The listing builds one solid part. Answer for the finished solid, in the listing's coordinates (mm). A direction names the side the tool comes from. Coordinates: 2 decimals unless noted, no trailing zeros. Loops run counter-clockwise (first coordinate to the right, second up) from the corner with the lowest first, then second, coordinate; pieces in that order, holes last. Notation, with made-up numbers: M 44,7 L 100,7 A30 cw 100,40 Z; hole C 33,-16.75 d2. An arc over 180 degrees is marked long. Answer as a JSON object with one key per item and string values. Group by question number.
1. A cutting plane is placed at C-C on y = 12. Give the vertices of the cut face in (x, z), and give its area (3 significant figures).
2. Straight lines are drawn through the part: L1, parallel to Y at x = 1.75, z = 0; L2, parallel to Z at x = -0.5, y = 17; L3, parallel to Y at x = 4.25, z = -0.5. For each, find the intervals that lie inside material, in ascending order.
3. A cutting plane is placed at D-D on y = -65. Give the vertices of the cut face in (x, z).
4. Given pin 1 (3 mm diameter, centred on y = -21.5, z = 3, fed in from +X); pin 2 (6 mm diameter, centred on x = 3.5, y = -49.5, fed in from -Z); pin 3 (2 mm diameter, centred on x = 4.5, y = 15, fed in from -Z), each flat-ended and moving along its own axis, determine where each tip first touches the part or whether it passes through.
5. Determine the mould class of faces 1 (the face through (0, -75, 0)), 2 (the face through (0, 26, 0)), 3 (the face through (-1.19, -27.12, -5.37)), 4 (the face through (0.054, -63.925, 1.686)) for opening direction Y: released by +Y, released by -Y, zero draft, split by the parting line, or undercut.
6. For faces 5 (the face through (-6.466, 10.353, -2.681)), 6 (the face through (-4, -55, -2)), determine the directions among +Z, -Z, +X, -X, +Y, -Y from which every point of the face is accessible in a straight line to the end or side of a thin tool.
7. A cutting plane is placed at A-A on z = 0. Give the vertices of the cut face in (x, y), and give its area (3 significant figures).
8. A cutting plane is placed at B-B on x = 0. Give the vertices of the cut face in (y, z).
from build123d import *

# Parameters (mm, degrees)
F0_R     = 5.5
F1_DEPTH = 75
F2_R     = 7
F3_DEPTH = 26
F4_SIZE2 = 0.437443
F4_SIZE  = 5
F5_R     = 5.5
F5_R_2   = 4
F6_DEPTH = 20
F7_R     = 2
F8_DEPTH = 12.5


with BuildPart() as f1:
    # F0 (on Front) → F1 (new body)
    with BuildSketch(Plane.XZ):
        Circle(F0_R)
    extrude(amount=F1_DEPTH)

    # F2 (on face) → F3 (join)
    with BuildSketch(Plane(origin=(0, 0, 0), x_dir=(-1, 0, 0), z_dir=(0, 1, 0))):
        Circle(F2_R)
    extrude(amount=F3_DEPTH)

    # F4
    f4_edges = [f1.edges().sort_by_distance(p)[0] for p in [
        (7, 26, 0),
    ]]
    chamfer(f4_edges, length=F4_SIZE, length2=F4_SIZE2)

    # F5 (on face) → F6 (cut)
    with BuildSketch(Plane.XZ.offset(75)):
        Circle(F5_R)
        Circle(F5_R_2, mode=Mode.SUBTRACT)
    extrude(amount=-F6_DEPTH, mode=Mode.SUBTRACT)

    # F7 (on Right) → F8 (cut, symmetric)
    with BuildSketch(Plane.YZ):
        with Locations((-65, 0)):
            Circle(F7_R)
    extrude(amount=F8_DEPTH, both=True, mode=Mode.SUBTRACT)


solid = f1.part
From the geometry:
{
 "1": {"outline": "C 0,0 d14", "area": "154 mm²"},
 "2": {"L1": "y = -75 to -67, -63 to 26", "L2": "z = -6.98 to 6.98", "L3": "y = -55 to 26"},
 "3": {"outline": "M -3.46,-2 A4 ccw 3.46,-2 Z; M -3.46,2 L 3.46,2 A4 ccw Z"},
 "4": {"pin 1": "stops at x = 5.29", "pin 2": "stops at z = -5.48", "pin 3": "stops at z = -6.06"},
 "5": {"face 1": "released by -Y", "face 2": "released by +Y", "face 3": "zero draft", "face 4": "undercut"},
 "6": {"face 5": "+Y, -Y", "face 6": "-Y"},
 "7": {"outline": "M -7,0 L -5.5,0 L -5.5,-55 L -4,-55 L -4,-63 L 4,-63 L 4,-55 L 5.5,-55 L 5.5,0 L 7,0 L 7,21 L 6.56,26 L -6.56,26 L -7,21 Z; M -4,-75 L 4,-75 L 4,-67 L -4,-67 Z", "area": "1,090 mm²"},
 "8": {"outline": "M -75,-4 L -55,-4 L -55,-5.5 L 0,-5.5 L 0,-7 L 21,-7 L 26,-6.56 L 26,6.56 L 21,7 L 0,7 L 0,5.5 L -55,5.5 L -55,4 L -75,4 Z; hole C -65,0 d4"}
}
